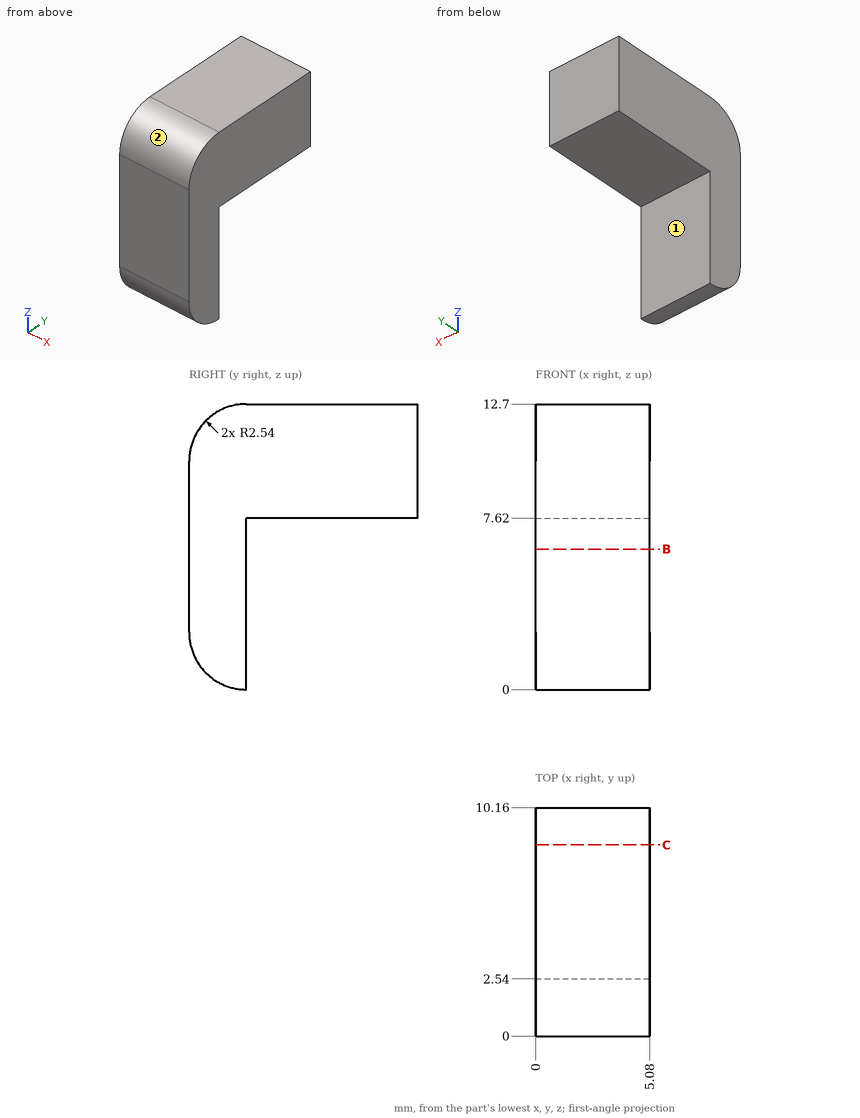
Geometry check sheet. Reference: drawing and pictorial views, mm from the part's lowest x, y, z. A direction names the side the tool comes from. Round coordinates to 2 decimals unless told otherwise and drop trailing zeros. Write each loop counter-clockwise with the first axis right and the second up, starting at its lowest first coordinate (ties: lowest second). Pieces come first, ordered by that corner, then holes. Notation, with made-up numbers: (-35, 50.25) -> (24, 50.25) arc R17 ccw to (24, 65.25) -> close; hole circle Ø10 at (-5.75, 6). An arc over 180 degrees is marked (long way). One line per question, with ' | ' between items. Start each with the question number.
1. Scan lines: line 1 along Z through (x, y) = (1.45, 7.75); line 2 along Y through (x, z) = (0.85, 4); line 3 along Z through (x, y) = (2.2, 1.5). Record each from-to range of solid material in increasing order. Write a range as from..to.
2. Set-up check for the marked faces 1 and 2: record each of +Z, -Z, +X, -X, +Y, -Y from which the full face is reachable in a straight line by a thin tool's end or side.
3. Depth check by flat-ended pin: pin 1 (2.5 mm diameter, centred on x = 4, y = 7.5, fed in from -Z); pin 2 (1 mm diameter, centred on x = 0.5, y = 1.5, fed in from -Z); pin 3 (1 mm diameter, centred on y = 2.5, z = 9.5, fed in from -X). Enter the tip coordinate at first touch or a pass-through.
4. Sectioned sample at C-C, the plane y = 8.5. Record the cut outline in (x, z), then the cut area to 3 significant figures.
5. Sectioned sample at B-B, the plane z = 6.25. Record the cut outline in (x, y), then the cut area to 3 significant figures.
Taken from the geometry:
1) line 1: z = 7.62..12.7 | line 2: y = 0..2.54 | line 3: z = 0.22..12.48
2) face 1: -Z, +X, -X, +Y | face 2: +Z, +X, -X, -Y
3) pin 1: stops at z = 7.62 | pin 2: stops at z = 0.06 | pin 3: stops at x = 0
4) outline: (0, 7.62) -> (5.08, 7.62) -> (5.08, 12.7) -> (0, 12.7) -> close | area: 25.8 mm^2
5) outline: (0, 0) -> (5.08, 0) -> (5.08, 2.54) -> (0, 2.54) -> close | area: 12.9 mm^2
